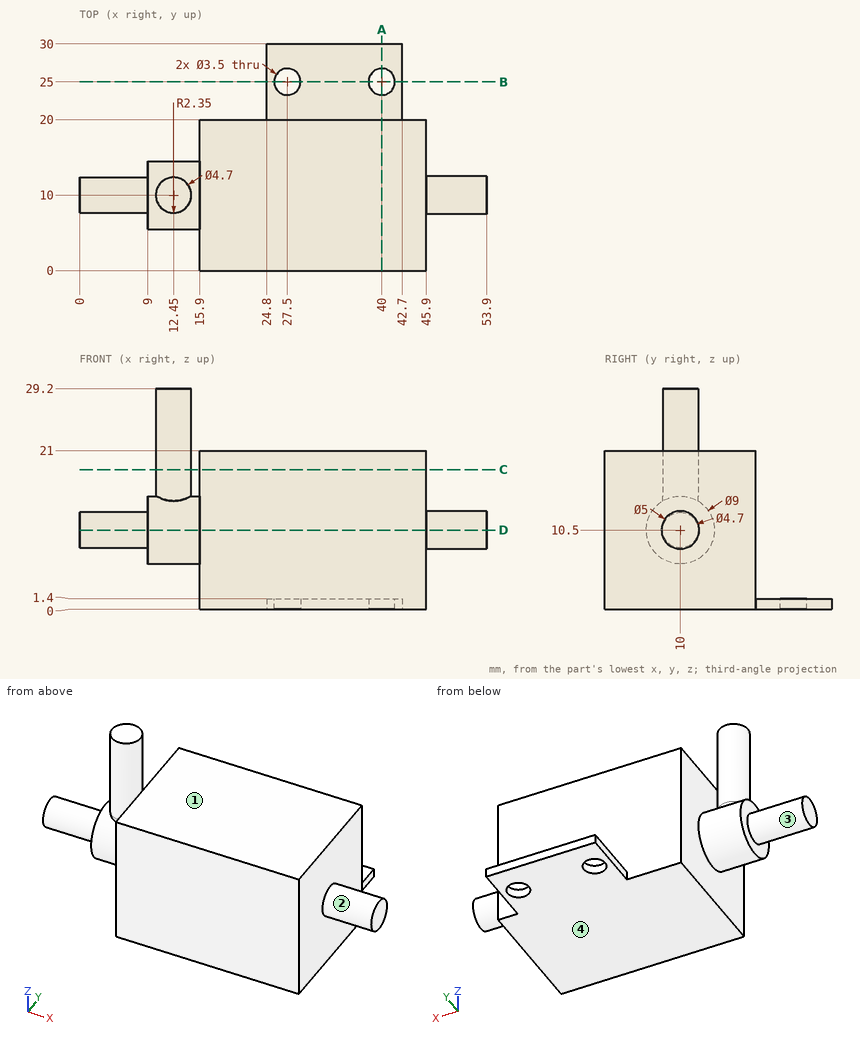
Study the drawing (mm; zero at the part's minimum x, y, z) and answer. A direction names the side the tool comes from. Give positions to 0.01 mm unless a question says otherwise; leave off trailing zeros. Order: outer loops, then holes, each group sorted by start corner. A loop starts at its lowest first (then second) coordinate and runs counter-clockwise, first axis right, second up. Notation, with made-up numbers: (87.5, 7.5) - (99.5, 7.5) arc R22 ccw to (99.5, 42.5) - close; hole circle Ø10 at (-12, 20). An arc over 180 degrees is marked (long way). Answer in a Markdown table with one row per item. Add a question column.
Q1. The part is cut by section D-D (z = 10.5). Determine the outline of the cut face in (x, y).
Q2. Find the intervals of material crossed by line 1 along Y through (x, z) = (40, 0.95); line 2 along Z through (x, y) = (45, 10.75); line 3 along Z through (x, y) = (36.5, 21.75), in increasing order. Write a range as [from, to].
Q3. The part is cut by section B-B (y = 25). Determine the outline of the cut face in (x, z), then the cut area to 3 significant figures.
Q4. Given P1, Ø2, axis at y = 15, z = 24.5, coming from the -X side; P2, Ø8, axis at x = 37.5, y = 23, coming from the +Z side; P3, Ø1.5, axis at x = 40, z = 21.5, coming from the -Y side; P4, Ø4, axis at x = 27.5, y = 25, coming from the +Z side, each flat-ended and moving along its own axis, determine where each tip first touches the part or whether it passes through.
Q5. The part is cut by section C-C (z = 18.5). Determine the outline of the cut face in (x, y).
Q6. Which of the six approach directions +Z, -Z, +X, -X, +Y, -Y give full straight-line access (tool end or side, diameter ignored) to the marked faces 1, 2, 3 and 4?
Q7. The part is cut by section A-A (x = 40). Determine the outline of the cut face in (y, z).
Determined:
| question | item | result |
|---|---|---|
| 1 | outline | (0, 7.65) - (9, 7.65) - (9, 5.5) - (15.9, 5.5) - (15.9, 0) - (45.9, 0) - (45.9, 7.5) - (53.9, 7.5) - (53.9, 12.5) - (45.9, 12.5) - (45.9, 20) - (15.9, 20) - (15.9, 14.5) - (9, 14.5) - (9, 12.35) - (0, 12.35) - close |
| 2 | line 1 | y = [0, 23.25], [26.75, 30] |
| 2 | line 2 | z = [0, 21] |
| 2 | line 3 | z = [0, 1.4] |
| 3 | outline | (24.8, 0) - (25.75, 0) - (25.75, 1.4) - (24.8, 1.4) - close; (29.25, 0) - (38.25, 0) - (38.25, 1.4) - (29.25, 1.4) - close; (41.75, 0) - (42.7, 0) - (42.7, 1.4) - (41.75, 1.4) - close |
| 3 | area | 15.3 mm² |
| 4 | P1 | passes through |
| 4 | P2 | stops at z = 21 |
| 4 | P3 | stops at y = 0 |
| 4 | P4 | stops at z = 1.4 |
| 5 | outline | circle Ø4.7 at (12.45, 10); (15.9, 0) - (45.9, 0) - (45.9, 20) - (15.9, 20) - close |
| 6 | face 1 | +Z, +X, +Y, -Y |
| 6 | face 2 | +X |
| 6 | face 3 | -X |
| 6 | face 4 | -Z, +X, -X, +Y, -Y |
| 7 | outline | (0, 0) - (23.25, 0) - (23.25, 1.4) - (20, 1.4) - (20, 21) - (0, 21) - close; (26.75, 0) - (30, 0) - (30, 1.4) - (26.75, 1.4) - close |
